Geometry check sheet. Reference: the model listing, model coordinates, mm. Give positions to 0.01 mm unless a question says otherwise; leave off trailing zeros. Use a Markdown table: item, result. Add a question column.
from build123d import *

# Parameters (mm, degrees)
SKETCH1_R           = 20
BOSS_EXTRUDE1_DEPTH = 3
CUT_EXTRUDE5_DEPTH  = 29.442925307
CIRPATTERN1_DEPTH   = 3


# Read off the part's stored shape, not the designer's step: CirPattern1
with BuildPart() as part:
    # Sketch1 → Boss-Extrude1 (new body)
    with BuildSketch(Plane.XY):
        Circle(SKETCH1_R)
    extrude(amount=BOSS_EXTRUDE1_DEPTH)

    # Sketch2 → Cut-Extrude5 (cut, through all)
    with BuildSketch(Plane.XY.offset(3)):
        Polygon((0.021198778, 19.999988765), (0.521152809, 19.993208841), (0.135577303, 9.997518193), align=None)
    extrude(amount=-CUT_EXTRUDE5_DEPTH, mode=Mode.SUBTRACT)


with BuildPart() as cut_extrude5_kept_piece:
    # of the separate pieces the step leaves, the one the design keeps (cut_extrude5_pieces_kept)
    add(part.part.solids().sort_by_distance((20, 0, 0))[0])

    # CirPattern1 outline → CirPattern1 (cut)
    with BuildSketch(Plane.XY):
        with BuildLine():
            Line((-3.107749756, 19.757071931), (-1.430048289, 9.895641117))
            Line((-1.430048289, 9.895641117), (-2.612890376, 19.828585521))
            ThreePointArc((-2.612890376, 19.828585521), (-2.860543555, 19.794375222), (-3.107749756, 19.757071931))
        make_face()
        with BuildLine():
            Line((1.697864531, 9.853223191), (3.642363483, 19.665533006))
            ThreePointArc((3.642363483, 19.665533006), (3.396259749, 19.709526119), (3.149625329, 19.750439499))
            Line((3.149625329, 19.750439499), (1.697864531, 9.853223191))
        make_face()
        with BuildLine():
            Line((3.2183447, 9.466309133), (6.673887081, 18.853626482))
            ThreePointArc((6.673887081, 18.853626482), (6.437695332, 18.935577073), (6.200497654, 19.014568864))
            Line((6.200497654, 19.014568864), (3.2183447, 9.466309133))
        make_face()
        with BuildLine():
            Line((4.659578542, 8.846303128), (9.541077431, 17.577481101))
            ThreePointArc((9.541077431, 17.577481101), (9.320613491, 17.695371275), (9.098693148, 17.810496438))
            Line((9.098693148, 17.810496438), (4.659578542, 8.846303128))
        make_face()
        with BuildLine():
            Line((5.986078095, 8.00847178), (12.17333479, 15.868519799))
            ThreePointArc((12.17333479, 15.868519799), (11.974027213, 16.019446707), (11.772848622, 16.167870479))
            Line((11.772848622, 16.167870479), (5.986078095, 8.00847178))
        make_face()
        with BuildLine():
            Line((7.165180539, 6.973445279), (14.505844245, 13.768822875))
            ThreePointArc((14.505844245, 13.768822875), (14.332600646, 13.949070196), (14.15711749, 14.127137891))
            Line((14.15711749, 14.127137891), (7.165180539, 6.973445279))
        make_face()
        with BuildLine():
            Line((8.167852459, 5.766709411), (16.481171674, 11.330091834))
            ThreePointArc((16.481171674, 11.330091834), (16.338257884, 11.535221282), (16.192791142, 11.73854828))
            Line((16.192791142, 11.73854828), (8.167852459, 5.766709411))
        make_face()
        with BuildLine():
            Line((8.969404743, 4.417978019), (18.050677958, 8.612376328))
            ThreePointArc((18.050677958, 8.612376328), (17.94161299, 8.837336935), (17.829744535, 9.060916653))
            Line((17.829744535, 9.060916653), (8.969404743, 4.417978019))
        make_face()
        with BuildLine():
            Line((9.550100515, 2.960461346), (19.175716644, 5.682595535))
            ThreePointArc((19.175716644, 5.682595535), (19.103186038, 5.921848023), (19.027670443, 6.160175186))
            Line((19.027670443, 6.160175186), (9.550100515, 2.960461346))
        make_face()
        with BuildLine():
            Line((9.895641117, 1.430048289), (19.828585545, 2.612890379))
            ThreePointArc((19.828585545, 2.612890379), (19.794375247, 2.860543558), (19.757071956, 3.10774976))
            Line((19.757071956, 3.10774976), (9.895641117, 1.430048289))
        make_face()
        with BuildLine():
            Line((9.997518193, -0.135577303), (19.993208862, -0.52115281))
            ThreePointArc((19.993208862, -0.52115281), (19.998161242, -0.271196982), (19.999988787, -0.021198778))
            Line((19.999988787, -0.021198778), (9.997518193, -0.135577303))
        make_face()
        with BuildLine():
            Line((9.853223191, -1.697864531), (19.665533023, -3.642363486))
            ThreePointArc((19.665533023, -3.642363486), (19.709526137, -3.396259752), (19.750439517, -3.149625332))
            Line((19.750439517, -3.149625332), (9.853223191, -1.697864531))
        make_face()
        with BuildLine():
            Line((9.466309133, -3.2183447), (18.853626494, -6.673887086))
            ThreePointArc((18.853626494, -6.673887086), (18.935577086, -6.437695337), (19.014568878, -6.200497658))
            Line((19.014568878, -6.200497658), (9.466309133, -3.2183447))
        make_face()
        with BuildLine():
            Line((8.846303128, -4.659578542), (17.577481109, -9.541077435))
            ThreePointArc((17.577481109, -9.541077435), (17.695371283, -9.320613495), (17.810496447, -9.098693153))
            Line((17.810496447, -9.098693153), (8.846303128, -4.659578542))
        make_face()
        with BuildLine():
            Line((8.00847178, -5.986078095), (15.868519802, -12.173334792))
            ThreePointArc((15.868519802, -12.173334792), (16.019446711, -11.974027216), (16.167870483, -11.772848624))
            Line((16.167870483, -11.772848624), (8.00847178, -5.986078095))
        make_face()
        with BuildLine():
            Line((6.973445279, -7.165180539), (13.768822874, -14.505844245))
            ThreePointArc((13.768822874, -14.505844245), (13.949070196, -14.332600646), (14.127137891, -14.15711749))
            Line((14.127137891, -14.15711749), (6.973445279, -7.165180539))
        make_face()
        with BuildLine():
            Line((5.766709411, -8.167852459), (11.330091831, -16.481171669))
            ThreePointArc((11.330091831, -16.481171669), (11.535221279, -16.33825788), (11.738548277, -16.192791138))
            Line((11.738548277, -16.192791138), (5.766709411, -8.167852459))
        make_face()
        with BuildLine():
            Line((4.417978019, -8.969404743), (8.612376324, -18.050677949))
            ThreePointArc((8.612376324, -18.050677949), (8.83733693, -17.941612981), (9.060916649, -17.829744526))
            Line((9.060916649, -17.829744526), (4.417978019, -8.969404743))
        make_face()
        with BuildLine():
            Line((2.960461346, -9.550100515), (5.682595531, -19.17571663))
            ThreePointArc((5.682595531, -19.17571663), (5.921848019, -19.103186025), (6.160175182, -19.02767043))
            Line((6.160175182, -19.02767043), (2.960461346, -9.550100515))
        make_face()
        with BuildLine():
            Line((1.430048289, -9.895641117), (2.612890376, -19.828585527))
            ThreePointArc((2.612890376, -19.828585527), (2.860543556, -19.794375229), (3.107749758, -19.757071938))
            Line((3.107749758, -19.757071938), (1.430048289, -9.895641117))
        make_face()
        with BuildLine():
            Line((-0.135577303, -9.997518193), (-0.521152809, -19.99320884))
            ThreePointArc((-0.521152809, -19.99320884), (-0.271196982, -19.99816122), (-0.021198778, -19.999988765))
            Line((-0.021198778, -19.999988765), (-0.135577303, -9.997518193))
        make_face()
        with BuildLine():
            Line((-1.697864531, -9.853223191), (-3.642363481, -19.665532998))
            ThreePointArc((-3.642363481, -19.665532998), (-3.396259748, -19.709526112), (-3.149625328, -19.750439493))
            Line((-3.149625328, -19.750439493), (-1.697864531, -9.853223191))
        make_face()
        with BuildLine():
            Line((-3.2183447, -9.466309133), (-6.673887077, -18.853626468))
            ThreePointArc((-6.673887077, -18.853626468), (-6.437695328, -18.93557706), (-6.20049765, -19.014568852))
            Line((-6.20049765, -19.014568852), (-3.2183447, -9.466309133))
        make_face()
        with BuildLine():
            Line((-4.659578542, -8.846303128), (-9.541077421, -17.577481083))
            ThreePointArc((-9.541077421, -17.577481083), (-9.320613482, -17.695371257), (-9.098693139, -17.810496421))
            Line((-9.098693139, -17.810496421), (-4.659578542, -8.846303128))
        make_face()
        with BuildLine():
            Line((-5.986078095, -8.00847178), (-12.173334774, -15.868519778))
            ThreePointArc((-12.173334774, -15.868519778), (-11.974027198, -16.019446687), (-11.772848606, -16.167870459))
            Line((-11.772848606, -16.167870459), (-5.986078095, -8.00847178))
        make_face()
        with BuildLine():
            Line((-7.165180539, -6.973445279), (-14.505844222, -13.768822853))
            ThreePointArc((-14.505844222, -13.768822853), (-14.332600623, -13.949070175), (-14.157117468, -14.127137869))
            Line((-14.157117468, -14.127137869), (-7.165180539, -6.973445279))
        make_face()
        with BuildLine():
            Line((-8.167852459, -5.766709411), (-16.481171644, -11.330091814))
            ThreePointArc((-16.481171644, -11.330091814), (-16.338257855, -11.535221261), (-16.192791114, -11.738548259))
            Line((-16.192791114, -11.738548259), (-8.167852459, -5.766709411))
        make_face()
        with BuildLine():
            Line((-8.969404743, -4.417978019), (-18.050677923, -8.612376311))
            ThreePointArc((-18.050677923, -8.612376311), (-17.941612955, -8.837336918), (-17.8297445, -9.060916636))
            Line((-17.8297445, -9.060916636), (-8.969404743, -4.417978019))
        make_face()
        with BuildLine():
            Line((-9.550100515, -2.960461346), (-19.175716604, -5.682595523))
            ThreePointArc((-19.175716604, -5.682595523), (-19.103185999, -5.921848011), (-19.027670404, -6.160175173))
            Line((-19.027670404, -6.160175173), (-9.550100515, -2.960461346))
        make_face()
        with BuildLine():
            Line((-9.895641117, -1.430048289), (-19.828585502, -2.612890373))
            ThreePointArc((-19.828585502, -2.612890373), (-19.794375204, -2.860543552), (-19.757071914, -3.107749754))
            Line((-19.757071914, -3.107749754), (-9.895641117, -1.430048289))
        make_face()
        with BuildLine():
            Line((-9.997518193, 0.135577303), (-19.993208819, 0.521152808))
            ThreePointArc((-19.993208819, 0.521152808), (-19.998161198, 0.271196981), (-19.999988743, 0.021198778))
            Line((-19.999988743, 0.021198778), (-9.997518193, 0.135577303))
        make_face()
        with BuildLine():
            Line((-9.853223191, 1.697864531), (-19.665532981, 3.642363478))
            ThreePointArc((-19.665532981, 3.642363478), (-19.709526095, 3.396259745), (-19.750439475, 3.149625326))
            Line((-19.750439475, 3.149625326), (-9.853223191, 1.697864531))
        make_face()
        with BuildLine():
            Line((-9.466309133, 3.2183447), (-18.853626455, 6.673887072))
            ThreePointArc((-18.853626455, 6.673887072), (-18.935577047, 6.437695323), (-19.014568838, 6.200497646))
            Line((-19.014568838, 6.200497646), (-9.466309133, 3.2183447))
        make_face()
        with BuildLine():
            Line((-8.846303128, 4.659578542), (-17.577481075, 9.541077417))
            ThreePointArc((-17.577481075, 9.541077417), (-17.695371249, 9.320613477), (-17.810496412, 9.098693135))
            Line((-17.810496412, 9.098693135), (-8.846303128, 4.659578542))
        make_face()
        with BuildLine():
            Line((-8.00847178, 5.986078095), (-15.868519775, 12.173334771))
            ThreePointArc((-15.868519775, 12.173334771), (-16.019446683, 11.974027195), (-16.167870455, 11.772848604))
            Line((-16.167870455, 11.772848604), (-8.00847178, 5.986078095))
        make_face()
        with BuildLine():
            Line((-6.973445279, 7.165180539), (-13.768822853, 14.505844223))
            ThreePointArc((-13.768822853, 14.505844223), (-13.949070175, 14.332600624), (-14.127137869, 14.157117468))
            Line((-14.127137869, 14.157117468), (-6.973445279, 7.165180539))
        make_face()
        with BuildLine():
            Line((-5.766709411, 8.167852459), (-11.330091817, 16.481171649))
            ThreePointArc((-11.330091817, 16.481171649), (-11.535221264, 16.338257859), (-11.738548262, 16.192791117))
            Line((-11.738548262, 16.192791117), (-5.766709411, 8.167852459))
        make_face()
        with BuildLine():
            Line((-4.417978019, 8.969404743), (-8.612376316, 18.050677932))
            ThreePointArc((-8.612376316, 18.050677932), (-8.837336922, 17.941612963), (-9.06091664, 17.829744508))
            Line((-9.06091664, 17.829744508), (-4.417978019, 8.969404743))
        make_face()
        with BuildLine():
            Line((-2.960461346, 9.550100515), (-5.682595527, 19.175716618))
            ThreePointArc((-5.682595527, 19.175716618), (-5.921848015, 19.103186012), (-6.160175178, 19.027670417))
            Line((-6.160175178, 19.027670417), (-2.960461346, 9.550100515))
        make_face()
    extrude(amount=CIRPATTERN1_DEPTH, mode=Mode.SUBTRACT)


solid = cut_extrude5_kept_piece.part
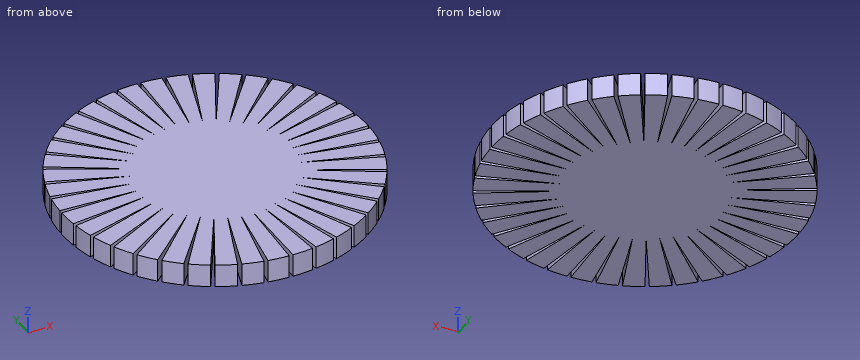
1) Gauge pin test, flat ends, axial feed: P1, Ø1.5, axis at x = -4, z = 1, coming from the +Y side; P2, Ø2, axis at x = 3.5, y = -5.5, coming from the -Z side. Record the tip position at first contact, or that the pin passes through.
2) Sectioned sample at A-A, the plane y = -10.5. Count the separate pieces of the cut face and the enclosed holes in it, and give its area (3 significant figures).
3) Material ranges on probe 1 along Y at (x, z) = (-18, 2.8); probe 2 along Y at (x, z) = (-1, 1.35), recorded low to high. Write a range as [from, to].
Check values:
| question | item | result |
|---|---|---|
| 1 | P1 | y = 19.73 |
| 1 | P2 | z = 0 |
| 2 | separate pieces | 14 |
| 2 | enclosed holes | 0 |
| 2 | area | 93.7 mm² |
| 3 | probe 1 | [-8.59, -5.81], [-5.35, -2.81], [-2.4, 0.04], [0.44, 2.89], [3.31, 5.88], [6.36, 8.72] |
| 3 | probe 2 | [-19.97, 19.97] |
